```python
from build123d import *

# Parameters (mm, degrees)
ESBO_O1_R                = 1.6
RESSALTO_EXTRUS_O1_DEPTH = 6


with BuildPart() as part:
    # Esboço1 → Ressalto-extrusão1 (new body)
    with BuildSketch(Plane.XZ.offset(6)):
        with BuildLine():
            Line((24.26036734, -24.5), (28.5, -24.5))
            ThreePointArc((28.5, -24.5), (31.122071197, -23.520718894), (32.460270003, -21.062371319))
            ThreePointArc((32.460270003, -21.062371319), (31.976417823, -19.646228266), (31.005959689, -18.507024557))
            Line((31.005959689, -18.507024557), (9.788591406, -1.452926582))
            ThreePointArc((9.788591406, -1.452926582), (9.894598333, -0.1563368), (9.829606895, 1.142954792))
            Line((9.829606895, 1.142954792), (10.623194285, 1.235230559))
            ThreePointArc((10.623194285, 1.235230559), (10.637816884, 1.237287137), (10.652472585, 1.239092776))
            add(Edge.make_bspline(
                [(10.652472585, 1.239092776), (12.4185109, 1.078975114), (14.239640851, 3.147417918)],
                knots=[0.078549619, 0.078549619, 0.078549619, 0.770539159, 0.770539159, 0.770539159], degree=2, weights=[1, 0.940738559, 1]))
            ThreePointArc((14.239640851, 3.147417918), (14.0864183, 3.774444408), (13.905599677, 4.394076552))
            add(Edge.make_bspline(
                [(13.905599677, 4.394076552), (11.294233474, 5.274835591), (9.84485826, 4.253150471)],
                knots=[5.512646149, 5.512646149, 5.512646149, 6.204635688, 6.204635688, 6.204635688], degree=2, weights=[1, 0.940738559, 1]))
            ThreePointArc((9.84485826, 4.253150471), (9.217248741, 4.230244905), (8.740864349, 4.639483569))
            ThreePointArc((8.740864349, 4.639483569), (8.570043058, 4.947916667), (8.388342806, 5.250068793))
            ThreePointArc((8.388342806, 5.250068793), (8.272123923, 5.86724911), (8.605765484, 6.399322114))
            add(Edge.make_bspline(
                [(8.605765484, 6.399322114), (10.21525836, 7.143675309), (10.758181759, 9.845564299)],
                knots=[0.078549619, 0.078549619, 0.078549619, 0.770539159, 0.770539159, 0.770539159], degree=2, weights=[1, 0.940738559, 1]))
            ThreePointArc((10.758181759, 9.845564299), (10.311973892, 10.311973892), (9.845564299, 10.758181759))
            add(Edge.make_bspline(
                [(9.845564299, 10.758181759), (7.143675309, 10.21525836), (6.399322114, 8.605765484)],
                knots=[2.371053495, 2.371053495, 2.371053495, 3.063043035, 3.063043035, 3.063043035], degree=2, weights=[1, 0.940738559, 1]))
            ThreePointArc((6.399322114, 8.605765484), (5.86724911, 8.272123923), (5.250068793, 8.388342806))
            ThreePointArc((5.250068793, 8.388342806), (4.947916667, 8.570043058), (4.639483569, 8.740864349))
            ThreePointArc((4.639483569, 8.740864349), (4.230244905, 9.217248741), (4.253150471, 9.84485826))
            add(Edge.make_bspline(
                [(4.253150471, 9.84485826), (5.274835591, 11.294233474), (4.394076552, 13.905599677)],
                knots=[0.078549619, 0.078549619, 0.078549619, 0.770539159, 0.770539159, 0.770539159], degree=2, weights=[1, 0.940738559, 1]))
            ThreePointArc((4.394076552, 13.905599677), (3.774444408, 14.0864183), (3.147417918, 14.239640851))
            add(Edge.make_bspline(
                [(3.147417918, 14.239640851), (1.078975114, 12.4185109), (1.239092776, 10.652472585)],
                knots=[2.371053495, 2.371053495, 2.371053495, 3.063043035, 3.063043035, 3.063043035], degree=2, weights=[1, 0.940738559, 1]))
            ThreePointArc((1.239092776, 10.652472585), (0.945124819, 10.097494016), (0.352521544, 9.889552362))
            ThreePointArc((0.352521544, 9.889552362), (0, 9.895833333), (-0.352521544, 9.889552362))
            ThreePointArc((-0.352521544, 9.889552362), (-0.945124819, 10.097494016), (-1.239092776, 10.652472585))
            add(Edge.make_bspline(
                [(-1.239092776, 10.652472585), (-1.078975114, 12.4185109), (-3.147417918, 14.239640851)],
                knots=[0.078549619, 0.078549619, 0.078549619, 0.770539159, 0.770539159, 0.770539159], degree=2, weights=[1, 0.940738559, 1]))
            ThreePointArc((-3.147417918, 14.239640851), (-3.774444408, 14.0864183), (-4.394076552, 13.905599677))
            add(Edge.make_bspline(
                [(-4.394076552, 13.905599677), (-5.274835591, 11.294233474), (-4.253150471, 9.84485826)],
                knots=[2.371053495, 2.371053495, 2.371053495, 3.063043035, 3.063043035, 3.063043035], degree=2, weights=[1, 0.940738559, 1]))
            ThreePointArc((-4.253150471, 9.84485826), (-4.230244905, 9.217248741), (-4.639483569, 8.740864349))
            ThreePointArc((-4.639483569, 8.740864349), (-4.947916667, 8.570043058), (-5.250068793, 8.388342806))
            ThreePointArc((-5.250068793, 8.388342806), (-5.86724911, 8.272123923), (-6.399322114, 8.605765484))
            add(Edge.make_bspline(
                [(-6.399322114, 8.605765484), (-7.143675309, 10.21525836), (-9.845564299, 10.758181759)],
                knots=[0.078549619, 0.078549619, 0.078549619, 0.770539159, 0.770539159, 0.770539159], degree=2, weights=[1, 0.940738559, 1]))
            ThreePointArc((-9.845564299, 10.758181759), (-10.311973892, 10.311973892), (-10.758181759, 9.845564299))
            add(Edge.make_bspline(
                [(-10.758181759, 9.845564299), (-10.21525836, 7.143675309), (-8.605765484, 6.399322114)],
                knots=[2.371053495, 2.371053495, 2.371053495, 3.063043035, 3.063043035, 3.063043035], degree=2, weights=[1, 0.940738559, 1]))
            ThreePointArc((-8.605765484, 6.399322114), (-8.272123923, 5.86724911), (-8.388342806, 5.250068793))
            ThreePointArc((-8.388342806, 5.250068793), (-8.570043058, 4.947916667), (-8.740864349, 4.639483569))
            ThreePointArc((-8.740864349, 4.639483569), (-9.217248741, 4.230244905), (-9.84485826, 4.253150471))
            add(Edge.make_bspline(
                [(-9.84485826, 4.253150471), (-11.294233474, 5.274835591), (-13.905599677, 4.394076552)],
                knots=[3.220142273, 3.220142273, 3.220142273, 3.912131812, 3.912131812, 3.912131812], degree=2, weights=[1, 0.940738559, 1]))
            ThreePointArc((-13.905599677, 4.394076552), (-14.0864183, 3.774444408), (-14.239640851, 3.147417918))
            add(Edge.make_bspline(
                [(-14.239640851, 3.147417918), (-12.4185109, 1.078975114), (-10.652472585, 1.239092776)],
                knots=[2.371053495, 2.371053495, 2.371053495, 3.063043035, 3.063043035, 3.063043035], degree=2, weights=[1, 0.940738559, 1]))
            ThreePointArc((-10.652472585, 1.239092776), (-10.557951639, 1.222896434), (-10.465816504, 1.196294788))
            ThreePointArc((-10.465816504, 1.196294788), (-10.466260875, 1.201681391), (-10.466707243, 1.207067829))
            Line((-10.466707243, 1.207067829), (-7.642065772, -0.272407964))
            Line((-7.642065772, -0.272407964), (21.127917729, -23.397147602))
            ThreePointArc((21.127917729, -23.397147602), (22.599906261, -24.216234622), (24.26036734, -24.5))
        make_face()
        Circle(ESBO_O1_R, mode=Mode.SUBTRACT)
        with Locations((22.598401843, -18.16414524)):
            Circle(ESBO_O1_R, mode=Mode.SUBTRACT)
    extrude(amount=-RESSALTO_EXTRUS_O1_DEPTH)


solid = part.part
```
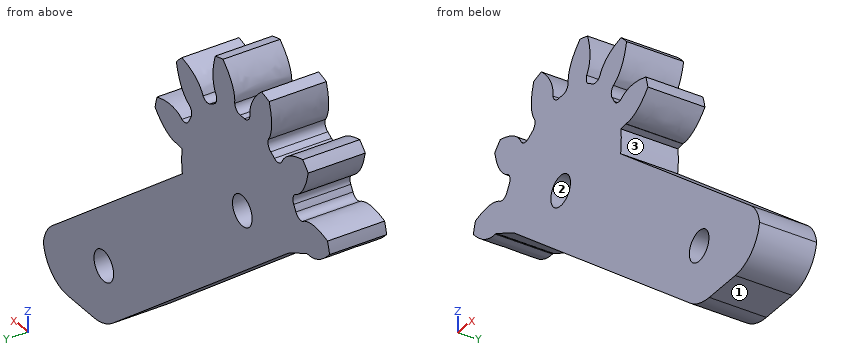
Part model, mm, in its own coordinate system. Face numbers are marked on the shaded views. Round coordinates to 2 decimals unless told otherwise and drop trailing zeros. Write each loop counter-clockwise with the first axis right and the second up, starting at its lowest first coordinate (ties: lowest second). Pieces come first, ordered by that corner, then holes.
Item 1: Cut at C-C, the plane x = 17. Give the cut face in (y, z), plus the area to 3 significant figures.
Results:
outline: (-6, -20.08) - (0, -20.08) - (0, -7.25) - (-6, -7.25) - close
area: 77.0 mm2
Item 2: Two-plate mould, pull along X, no slides. Class the marked faces 1, 2 and 3: +X half, -X half, draft (parallel to the pull), parting line (faces both ways), or undercut.
Results:
face 1: draft
face 2: undercut
face 3: +X half
Item 3: Cut at A-A, the plane z = -15.5. Give the cut face in (x, y).
Results:
outline: (11.3, -6) - (27.26, -6) - (27.26, 0) - (11.3, 0) - close
Item 4: Drop flat-ended pins along their axis: pin 1 Ø1 at (x, y) = (8.5, -2) entering from -Z; pin 2 Ø10 at (x, z) = (13, -10) entering from +Y; pin 3 Ø1 at (x, y) = (-7.5, -1.5) entering from +Z; pin 4 Ø3 at (y, z) = (-3, -1.5) entering from -X. Give the stop position or say it passes through.
Results:
pin 1: stops at z = -13.65
pin 2: stops at y = 0
pin 3: stops at z = 10.14
pin 4: stops at x = -8.16
Item 5: Probe L1, parallel to Z at x = 0, y = -2.6; L2, parallel to X at y = -4.5, z = 0.5; L3, parallel to X at y = -4.5, z = -19.5. List the from-to ranges inside material, lowest first.
Results:
L1: z = -6.41 to -1.6, 1.6 to 9.9
L2: x = -9.12 to -1.52, 1.52 to 9.88
L3: x = 16.28 to 21.72, 23.48 to 31.89
Item 6: Cut at B-B, the plane y = -5.5. Count the separate pieces of the cut face and the enclosed holes in it, plus the area to 3 significant figures.
Results:
separate pieces: 1
enclosed holes: 2
area: 594 mm2
